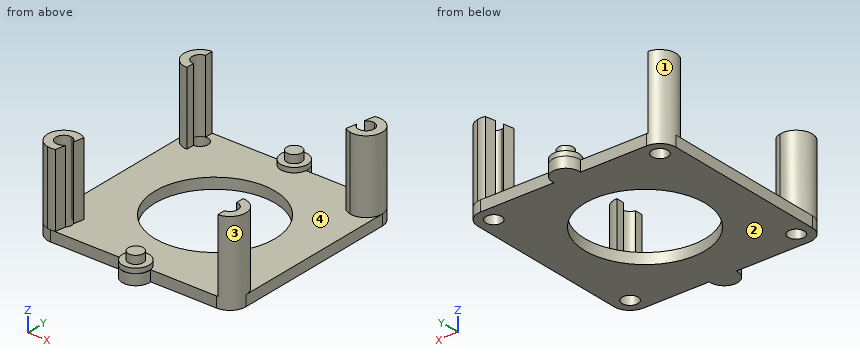
from build123d import *

# Parameters (mm, degrees)
SKETCH1_R      = 1.5
SKETCH1_R_2    = 11.2
EXTRUDE1_DEPTH = 2
SKETCH2_R      = 2.5
EXTRUDE2_DEPTH = 0.9
SKETCH3_R      = 1.4
EXTRUDE3_DEPTH = 1.5
EXTRUDE4_DEPTH = 13.5
EXTRUDE5_DEPTH = 13.5
SKETCH6_W      = 0.2
SKETCH6_H      = 4.339086574
EXTRUDE6_DEPTH = 13.5


with BuildPart() as part:
    # Sketch1 → Extrude1 (new body)
    with BuildSketch(Plane.XY):
        with BuildLine():
            Line((-18.5, 15.5), (-18.5, -15.5))
            ThreePointArc((-18.5, -15.5), (-17.621320344, -17.621320344), (-15.5, -18.5))
            Line((-15.5, -18.5), (-1.853762559, -18.5))
            ThreePointArc((-1.853762559, -18.5), (0.656979507, -21.34366179), (3.167721572, -18.5))
            Line((3.167721572, -18.5), (15.5, -18.5))
            ThreePointArc((15.5, -18.5), (17.621320344, -17.621320344), (18.5, -15.5))
            Line((18.5, -15.5), (18.5, 15.5))
            ThreePointArc((18.5, 15.5), (17.621320344, 17.621320344), (15.5, 18.5))
            Line((15.5, 18.5), (1.819299557, 18.5))
            ThreePointArc((1.819299557, 18.5), (-0.656979507, 21.309467878), (-3.13325857, 18.5))
            Line((-3.13325857, 18.5), (-15.5, 18.5))
            ThreePointArc((-15.5, 18.5), (-17.621320344, 17.621320344), (-18.5, 15.5))
        make_face()
        with Locations((15.5, 15.5)):
            Circle(SKETCH1_R, mode=Mode.SUBTRACT)
        with Locations((-15.5, 15.5)):
            Circle(SKETCH1_R, mode=Mode.SUBTRACT)
        Circle(SKETCH1_R_2, mode=Mode.SUBTRACT)
        with Locations((15.5, -15.5)):
            Circle(SKETCH1_R, mode=Mode.SUBTRACT)
        with Locations((-15.5, -15.5)):
            Circle(SKETCH1_R, mode=Mode.SUBTRACT)
    extrude(amount=EXTRUDE1_DEPTH)

    # Sketch2 → Extrude2 (add)
    with BuildSketch(Plane.XY.offset(2)):
        with Locations(Location((-0.656979507, 18.813431552, 0), (0, 0, 187.202274666))):
            Circle(SKETCH2_R)
        with Locations(Location((0.656979507, -18.813431552, 0), (0, 0, 180))):
            Circle(SKETCH2_R)
    extrude(amount=EXTRUDE2_DEPTH)

    # Sketch3 → Extrude3 (add)
    with BuildSketch(Plane.XY.offset(2.9)):
        with Locations((-0.656979507, 18.813431552)):
            Circle(SKETCH3_R)
        with Locations((0.656979507, -18.813431552)):
            Circle(SKETCH3_R)
    extrude(amount=EXTRUDE3_DEPTH)

    # Sketch4 → Extrude4 (add)
    with BuildSketch(Plane.XY.offset(2)):
        with BuildLine():
            Line((15.5, -14), (15.5, -12.5))
            ThreePointArc((15.5, -12.5), (18.5, -15.5), (15.5, -18.5))
            Line((15.5, -18.5), (15.5, -17))
            ThreePointArc((15.5, -17), (17, -15.5), (15.5, -14))
        make_face()
        with BuildLine():
            Line((-14.897310813, -12.561162518), (-15.198655407, -14.030581259))
            ThreePointArc((-15.198655407, -14.030581259), (-16.969418741, -15.198655407), (-15.801344593, -16.969418741))
            Line((-15.801344593, -16.969418741), (-16.102689187, -18.438837482))
            ThreePointArc((-16.102689187, -18.438837482), (-18.438837482, -14.897310813), (-14.897310813, -12.561162518))
        make_face()
        with BuildLine():
            Line((-15.5, 17), (-15.5, 18.5))
            ThreePointArc((-15.5, 18.5), (-18.5, 15.5), (-15.5, 12.5))
            Line((-15.5, 12.5), (-15.5, 14))
            ThreePointArc((-15.5, 14), (-17, 15.5), (-15.5, 17))
        make_face()
        with BuildLine():
            Line((16.102689187, 18.438837482), (15.801344593, 16.969418741))
            ThreePointArc((15.801344593, 16.969418741), (16.969418741, 15.198655407), (15.198655407, 14.030581259))
            Line((15.198655407, 14.030581259), (14.897310813, 12.561162518))
            ThreePointArc((14.897310813, 12.561162518), (18.438837482, 14.897310813), (16.102689187, 18.438837482))
        make_face()
    extrude(amount=EXTRUDE4_DEPTH)

    # Sketch5 → Extrude5 (add)
    with BuildSketch(Plane.XY.offset(15.5)):
        with BuildLine():
            Line((14.684749395, 18.387103471), (14.348199746, 16.460914239))
            ThreePointArc((14.348199746, 16.460914239), (16.977615135, 15.241826583), (14.090600687, 14.98658635))
            Line((14.090600687, 14.98658635), (13.754051037, 13.060397118))
            ThreePointArc((13.754051037, 13.060397118), (18.45523027, 14.983653166), (14.684749395, 18.387103471))
        make_face()
        with BuildLine():
            Line((-13.754051037, -13.060397118), (-14.090600687, -14.98658635))
            ThreePointArc((-14.090600687, -14.98658635), (-16.977615135, -15.241826583), (-14.348199746, -16.460914239))
            Line((-14.348199746, -16.460914239), (-14.684749395, -18.387103471))
            ThreePointArc((-14.684749395, -18.387103471), (-18.45523027, -14.983653166), (-13.754051037, -13.060397118))
        make_face()
    extrude(amount=-EXTRUDE5_DEPTH)

    # Sketch6 → Extrude6 (cut)
    with BuildSketch(Plane.XY.offset(15.5)):
        Polygon((-15.5, 19.617766956), (-15.5, 15.861892736), (-15.7, 15.875), (-15.7, 19.617766956), align=None)
        with Locations((15.6, -18.094430424)):
            Rectangle(SKETCH6_W, SKETCH6_H)
    extrude(amount=-EXTRUDE6_DEPTH, mode=Mode.SUBTRACT)


solid = part.part
Design review of the part built by this model. Coordinates are the model's own, in mm. Face numbers are marked on the shaded views. A direction names the side the tool comes from. Give positions to 0.01 mm unless a question says otherwise; leave off trailing zeros. Write each loop counter-clockwise with the first axis right and the second up, starting at its lowest first coordinate (ties: lowest second). Pieces come first, ordered by that corner, then holes. Notation, with made-up numbers: M -21,-28 L 4,-28 A4 ccw 4,-23 Z; hole C 27,-7 d11. An arc over 180 degrees is marked long. Answer as a JSON object with one key per item and string values. Group by question number.
1) We need section D-D (y = 14.5). Give the boundary of the cut face in (x, z).
2) We need section B-B (z = 1.5). Give the boundary of the cut face in (x, y).
3) We need section A-A (y = 0). Give the boundary of the cut face in (x, z), and give its area (3 significant figures).
4) Tool access review of the marked faces 1, 2, 3 and 4: name each direction out of +Z, -Z, +X, -X, +Y, -Y from which nothing blocks a thin tool from reaching the whole face with its end or side.
5) For line 1 along Y through (x, z) = (-15.5, 1.2); line 2 along Y through (x, z) = (-12, 1), list the stretches that pass through material, from the lowest coordinate up.
6) We need section C-C (x = 5). Give the boundary of the cut face in (y, z).
7) Clearance check with flat-ended pins moving along their axes: pin 1 Ø1.8 at (x, y) = (15.5, 15.5) entering from +Z; pin 2 Ø0.8 at (x, y) = (0.5, 20.5) entering from -Z; pin 3 Ø2 at (x, z) = (11.5, 1) entering from +Y; pin 4 Ø1.2 at (y, z) = (13, 7) entering from +X. State where each tip first meets the part, or that it passes through.
Answer key:
{
 "1": {"outline": "M -18.5,0 L -16.62,0 L -16.62,15.5 L -18.33,15.5 L -18.33,2 L -18.5,2 Z; M -14.38,0 L 14.38,0 L 14.38,15.5 L 14.01,15.5 L 14.01,2 L -14.38,2 Z; M 16.62,0 L 18.5,0 L 18.5,2 L 18.33,2 L 18.33,15.5 L 16.62,15.5 Z"},
 "2": {"outline": "M -18.5,-15.5 A3 ccw -15.5,-18.5 L -1.85,-18.5 A2.53 ccw long 3.17,-18.5 L 15.5,-18.5 A3 ccw 18.5,-15.5 L 18.5,15.5 A3 ccw 15.5,18.5 L 1.82,18.5 A2.5 ccw long -3.13,18.5 L -15.5,18.5 A3 ccw -18.5,15.5 Z; hole C -15.5,-15.5 d3; hole C -15.5,15.5 d3; hole C 0,0 d22.4; hole C 15.5,-15.5 d3; hole C 15.5,15.5 d3"},
 "3": {"outline": "M -18.5,0 L -11.2,0 L -11.2,2 L -18.5,2 Z; M 11.2,0 L 18.5,0 L 18.5,2 L 11.2,2 Z", "area": "29.2 mm²"},
 "4": {"face 1": "+Z, -X", "face 2": "-Z, +X, -X, +Y, -Y", "face 3": "+Z, +X", "face 4": "+Z"},
 "5": {"line 1": "y = -18.5 to -17, -14 to 14, 17 to 18.5", "line 2": "y = -18.5 to 18.5"},
 "6": {"outline": "M -18.5,0 L -10.02,0 L -10.02,2 L -18.5,2 Z; M 10.02,0 L 18.5,0 L 18.5,2 L 10.02,2 Z"},
 "7": {"pin 1": "passes through", "pin 2": "stops at z = 0", "pin 3": "stops at y = 18.5", "pin 4": "stops at x = 17.82"}
}
